Design review of the part built by this model. Coordinates are the model's own, in mm. A direction names the side the tool comes from. Round coordinates to 2 decimals unless told otherwise and drop trailing zeros. Order: outer loops, then holes, each group sorted by start corner. A loop starts at its lowest first (then second) coordinate and runs counter-clockwise, first axis right, second up.
from build123d import *

# Parameters (mm, degrees)
F0_W      = 100
F0_H      = 60
F0_R      = 1.5
F1_DEPTH  = 1.55
F2_W      = 17
F2_H      = 16
F2_W_2    = 4
F3_DEPTH  = 13.5
F4_W      = 14.8
F4_H      = 16.5
F4_H_2    = 0.8
F5_DEPTH  = 16
F6_W      = 47.7
F6_H      = 4
F7_DEPTH  = 2
F8_W      = 17
F8_H      = 6.5
F9_DEPTH  = 8
F10_W     = 11
F10_H     = 15
F10_W_2   = 1
F11_DEPTH = 6
F12_W     = 6.3
F12_H     = 2
F13_DEPTH = 11
F14_W     = 12
F14_H     = 5
F15_DEPTH = 11
F17_DEPTH = 11
F19_DEPTH = 12


with BuildPart() as f1:
    # F0 (on Top) → F1 (new body)
    with BuildSketch(Plane.XY):
        Rectangle(F0_W, F0_H)
        with Locations((-27.5, -26.5)):
            Circle(F0_R, mode=Mode.SUBTRACT)
        with Locations((46.5, -26.5)):
            Circle(F0_R, mode=Mode.SUBTRACT)
        with Locations((-27.5, 26.5)):
            Circle(F0_R, mode=Mode.SUBTRACT)
        with Locations((46.5, 26.5)):
            Circle(F0_R, mode=Mode.SUBTRACT)
    extrude(amount=F1_DEPTH)

    # F2 (on face) → F3 (join)
    with BuildSketch(Plane.XY.offset(1.55)):
        with Locations((41.5, -14.5)):
            Rectangle(F2_W, F2_H)
        with Locations((52, -14.5)):
            Rectangle(F2_W_2, F2_H)
    extrude(amount=F3_DEPTH)

    # F4 (on face) → F5 (join)
    with BuildSketch(Plane.XY.offset(1.55)):
        with Locations((-13.9, -21.75)):
            Rectangle(F4_W, F4_H)
        with Locations((-13.9, -30.4)):
            Rectangle(F4_W, F4_H_2)
    extrude(amount=F5_DEPTH)

    # F6 (on face) → F7 (join)
    with BuildSketch(Plane(origin=(0, 0, 0), x_dir=(1, 0, 0), z_dir=(0, 0, -1))):
        with Locations((19.15, 26.5)):
            Rectangle(F6_W, F6_H)
        with Locations((19.15, -26.5)):
            Rectangle(F6_W, F6_H)
    extrude(amount=F7_DEPTH)

    # F8 (on face) → F9 (join)
    with BuildSketch(Plane.XY.offset(1.55)):
        with Locations((-15, 26.55)):
            Rectangle(F8_W, F8_H)
    extrude(amount=F9_DEPTH)

    # F10 (on face) → F11 (join)
    with BuildSketch(Plane.XY.offset(1.55)):
        with Locations((-44.5, -2.5)):
            Rectangle(F10_W, F10_H)
        with Locations((-50.5, -2.5)):
            Rectangle(F10_W_2, F10_H)
    extrude(amount=F11_DEPTH)

    # F12 (on face) → F13 (cut)
    with BuildSketch(Plane.YZ.offset(54)):
        Polygon((-8.5, 12.55), (-20.5, 12.55), (-20.5, 5.55), (-17.6502, 5.55), (-11.3502, 5.55), (-8.5, 5.55), align=None)
        with Locations((-14.5002, 4.55)):
            Rectangle(F12_W, F12_H)
    extrude(amount=-F13_DEPTH, mode=Mode.SUBTRACT)

    # F14 (on face) → F15 (cut)
    with BuildSketch(Plane.XZ.offset(30.8)):
        with Locations((-13.8, 12.55)):
            Rectangle(F14_W, F14_H)
        with Locations((-13.8, 5.55)):
            Rectangle(F14_W, F14_H)
    extrude(amount=-F15_DEPTH, mode=Mode.SUBTRACT)

    # F16 (on face) → F17 (cut)
    with BuildSketch(Plane(origin=(-51, 0, 0), x_dir=(0, -1, 0), z_dir=(-1, 0, 0))):
        Polygon((8.5, 6.35), (-3.5, 6.35), (-1.5, 2.85), (6.5, 2.85), align=None)
    extrude(amount=-F17_DEPTH, mode=Mode.SUBTRACT)

    # F18 (on face) → F19 (cut, through all)
    with BuildSketch(Plane(origin=(-51, 0, 0), x_dir=(0, -1, 0), z_dir=(-1, 0, 0))):
        Polygon((10, 6.064864339), (7.4200775205, 1.55), (10, 1.55), align=None)
        Polygon((-5, 1.55), (-2.4200775205, 1.55), (-5, 6.064864339), align=None)
    extrude(amount=-F19_DEPTH, mode=Mode.SUBTRACT)


solid = f1.part
1) Clearance check with flat-ended pins moving along their axes: P1, Ø4, axis at x = -19.5, z = 9.5, coming from the +Y side; P2, Ø5, axis at x = 35.5, y = -20.5, coming from the +Z side; P3, Ø0.8, axis at y = -9.5, z = 0.5, coming from the +X side. State where each tip first meets the part, or that it passes through.
Results:
P1: stops at y = 29.8
P2: stops at z = 15.05
P3: stops at x = 50
2) To check wall thickness, follow line 1 along Y through (x, z) = (46.5, 0.3); line 2 along X through (y, z) = (-17, 14.25); line 3 along Y through (x, z) = (47.5, 4.5). State the ranges of each line that lie inside material, in increasing order.
Results:
line 1: y = -30 to -28, -25 to 25, 28 to 30
line 2: x = -21.3 to -6.5, 33 to 54
line 3: y = -22.5 to -17.65, -11.35 to -6.5
3) Take a section at C-C on x = -27.5. Give the boundary of the cut face in (y, z).
Results:
outline: (-30, 0) - (-28, 0) - (-28, 1.55) - (-30, 1.55) - close; (-25, 0) - (25, 0) - (25, 1.55) - (-25, 1.55) - close; (28, 0) - (30, 0) - (30, 1.55) - (28, 1.55) - close
4) Take a section at B-B on y = -26.5. Give the boundary of the cut face in (x, z), plus the area to 3 significant figures.
Results:
outline: (-50, 0) - (-29, 0) - (-29, 1.55) - (-50, 1.55) - close; (-26, 0) - (-4.7, 0) - (-4.7, -2) - (43, -2) - (43, 0) - (45, 0) - (45, 1.55) - (-6.5, 1.55) - (-6.5, 17.55) - (-21.3, 17.55) - (-21.3, 1.55) - (-26, 1.55) - close; (48, 0) - (50, 0) - (50, 1.55) - (48, 1.55) - close; hole (-19.8, 3.05) - (-7.8, 3.05) - (-7.8, 8.05) - (-19.8, 8.05) - close; hole (-19.8, 10.05) - (-7.8, 10.05) - (-7.8, 15.05) - (-19.8, 15.05) - close
area: 358 mm2
5) The part is to be moulded in two halves that separate along Z. For faces 1 (the face through (-45.084, 3.692, 3.776)), 2 (the face through (-21.3, -22, 9)), 3 (the face through (43, -14, 15.05)), say which applies: released by +Z, released by -Z, zero draft, split by the parting line, or undercut.
Results:
face 1: undercut
face 2: zero draft
face 3: released by +Z
6) Take a section at D-D on y = 26.5. Give the boundary of the cut face in (x, z), plus the area to 3 significant figures.
Results:
outline: (-50, 0) - (-29, 0) - (-29, 1.55) - (-50, 1.55) - close; (-26, 0) - (-4.7, 0) - (-4.7, -2) - (43, -2) - (43, 0) - (45, 0) - (45, 1.55) - (-6.5, 1.55) - (-6.5, 9.55) - (-23.5, 9.55) - (-23.5, 1.55) - (-26, 1.55) - close; (48, 0) - (50, 0) - (50, 1.55) - (48, 1.55) - close
area: 377 mm2
7) For faces 4 (the face through (-14, -19.8, 13)), 5 (the face through (-15, 29.8, 5)), 6 (the face through (-14, -13.5, 9)), 7 (the face through (49, -19, 5.55)), list the 3-axis set-ups (+Z, -Z, +X, -X, +Y, -Y) from which the entire face can be reached by the end or side of a thin tool; tool diameter is ignored.
Results:
face 4: -Y
face 5: +Z, +X, -X, +Y
face 6: +Z, -X
face 7: +X
8) Take a section at A-A on x = 46.5. Give the boundary of the cut face in (y, z).
Results:
outline: (-30, 0) - (-28, 0) - (-28, 1.55) - (-30, 1.55) - close; (-25, 0) - (25, 0) - (25, 1.55) - (-6.5, 1.55) - (-6.5, 15.05) - (-22.5, 15.05) - (-22.5, 1.55) - (-25, 1.55) - close; (28, 0) - (30, 0) - (30, 1.55) - (28, 1.55) - close; hole (-20.5, 5.55) - (-17.65, 5.55) - (-17.65, 3.55) - (-11.35, 3.55) - (-11.35, 5.55) - (-8.5, 5.55) - (-8.5, 12.55) - (-20.5, 12.55) - close
